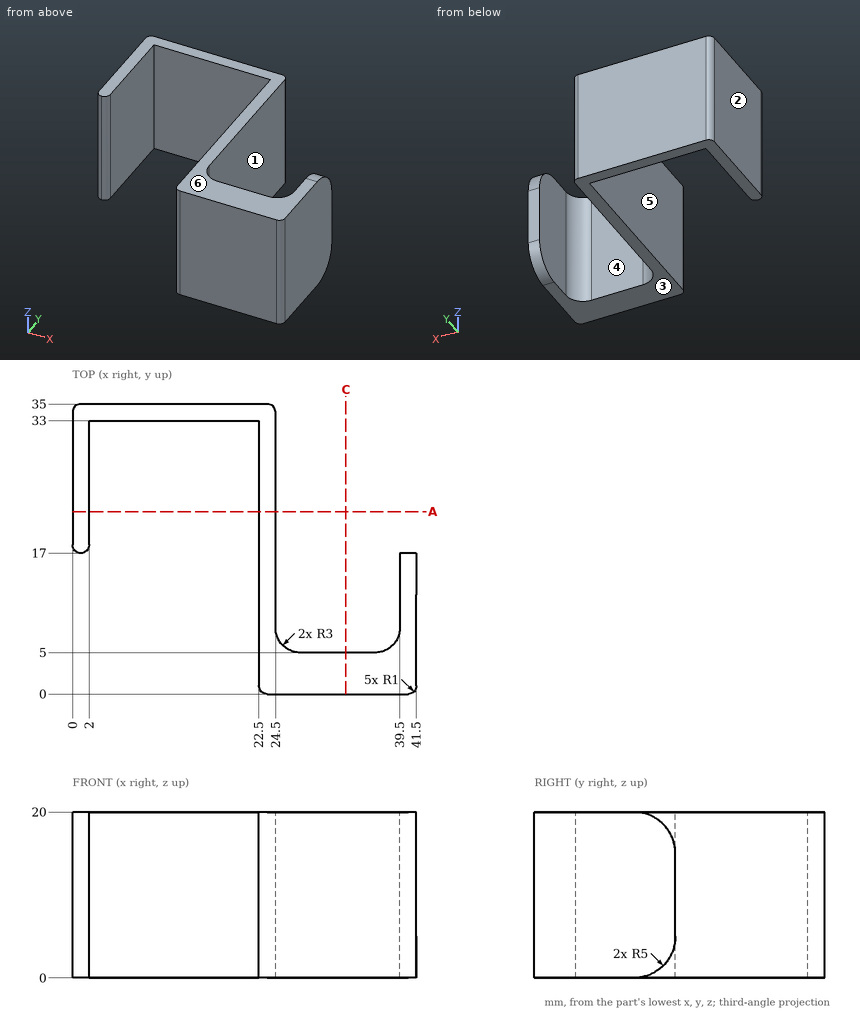
Geometry check sheet. Reference: drawing and pictorial views, mm from the part's lowest x, y, z. A direction names the side the tool comes from. Round coordinates to 2 decimals unless told otherwise and drop trailing zeros. Loops run counter-clockwise (first coordinate to the right, second up) from the corner with the lowest first, then second, coordinate; pieces in that order, holes last. Notation, with made-up numbers: (75.25, -17) - (134.25, -17) arc R8 cw to (134.25, -12) - close; hole circle Ø10 at (-31.75, 40.25). An arc over 180 degrees is marked (long way). Answer in a Markdown table with one row per item. Add a question column.
Q1. Material ranges on line 1 (X direction, y = 10.5, z = 2.5); line 2 (X direction, y = 27, z = 11.5); line 3 (Y direction, x = 3, z = 15), recorded low to high.
Q2. Tool access check on the marked faces 4, 5 and 6. Record the directions out of +Z, -Z, +X, -X, +Y, -Y that give a thin tool (end or side, any length) a straight path to the whole face; none if there is none.
Q3. Gauge pin test, flat ends, axial feed: pin 1 (2.5 mm diameter, centred on x = 32.5, z = 14.5, fed in from +Y); pin 2 (1 mm diameter, centred on y = 18.5, z = 15, fed in from +X); pin 3 (2 mm diameter, centred on y = 8, z = 6.5, fed in from -X). Record the tip position at first contact, or that the pin passes through.
Q4. Section check A-A on y = 22. Enter the section's corners in (x, z), plus the area to 3 significant figures.
Q5. Release check for a two-part mould opening along X. For the marked faces 1, 2 and 3 record: pulls with the +X half, pulls with the -X half, needs draft (parallel to the pull), parting line crosses it, or undercut.
Q6. Section check C-C on x = 33. Enter the section's corners in (y, z), plus the area to 3 significant figures.
Found:
| question | item | result |
|---|---|---|
| 1 | line 1 | x = 22.5 to 24.5, 39.5 to 41.5 |
| 1 | line 2 | x = 0 to 2, 22.5 to 24.5 |
| 1 | line 3 | y = 33 to 35 |
| 2 | face 4 | +Z, -Z, +Y |
| 2 | face 5 | +Z, -Z, -Y |
| 2 | face 6 | +Z, +X, -X, +Y, -Y |
| 3 | pin 1 | stops at y = 5 |
| 3 | pin 2 | stops at x = 24.5 |
| 3 | pin 3 | stops at x = 22.5 |
| 4 | outline | (0, 0) - (2, 0) - (2, 20) - (0, 20) - close; (22.5, 0) - (24.5, 0) - (24.5, 20) - (22.5, 20) - close |
| 4 | area | 80.0 mm² |
| 5 | face 1 | undercut |
| 5 | face 2 | pulls with the -X half |
| 5 | face 3 | needs draft |
| 6 | outline | (0, 0) - (5, 0) - (5, 20) - (0, 20) - close |
| 6 | area | 100 mm² |
